from build123d import *

# Parameters (mm, degrees)
F0_W     = 30
F0_H     = 10
F0_R     = 2.75
F1_DEPTH = 7
F3_DEPTH = 15
F4_R     = 3
F5_R     = 1.5
F6_DEPTH = 25


# Not quite as in the source:
# - a feature names something its author has since deleted; it is built from what else it names


with BuildPart() as f1:
    # F0 (on Top) → F1 (new body)
    with BuildSketch(Plane.XY):
        with Locations((-23.3256115019, 35.3867347538)):
            Rectangle(F0_W, F0_H)
        with Locations((-32.3030129075, 35.3867347538)):
            Circle(F0_R, mode=Mode.SUBTRACT)
    extrude(amount=F1_DEPTH)

    # F2 (on face) → F3 (join)
    with BuildSketch(Plane.YZ.offset(-8.3256115019)):
        Polygon((30.3867347538, -10), (40.3867347538, 0), (30.3867347538, 0), align=None)
        Polygon((40.3867347538, 7), (40.3867347538, 0), (47.3867347538, 7), align=None)
    extrude(amount=-F3_DEPTH)

    # F4
    f4_edges = [f1.edges().sort_by_distance(p)[0] for p in [
        (-38.325612, 40.386735, 3.5),
        (-38.325612, 30.386735, 3.5),
    ]]
    fillet(f4_edges, radius=F4_R)

    # F5 (on face) → F6 (cut)
    with BuildSketch(Plane(origin=(0, 20.1933673769, -20.1933673769), x_dir=(1, 0, 0), z_dir=(0, 0.7071067812, -0.7071067812))):
        with Locations((-15.8256115019, -35.0243411958)):
            Circle(F5_R)
    extrude(amount=-F6_DEPTH, mode=Mode.SUBTRACT)


solid = f1.part
Geometry check sheet. Reference: the model listing, model coordinates, mm. A direction names the side the tool comes from. Give positions to 0.01 mm unless a question says otherwise; leave off trailing zeros. Order: outer loops, then holes, each group sorted by start corner. A loop starts at its lowest first (then second) coordinate and runs counter-clockwise, first axis right, second up. Notation, with made-up numbers: (40.5, 17) - (78.5, 17) arc R16 ccw to (78.5, 38) - close; hole circle Ø8 at (-33.5, -35). An arc over 180 degrees is marked (long way). Answer as a JSON object with one key per item and string values.
(1) Cross-section at C-C (z = 1.25). Record the cut outline in (x, y), then the cut area to 3 significant figures.
Report:
{"outline": "(-38.33, 33.39) arc R3 ccw to (-35.33, 30.39) - (-8.33, 30.39) - (-8.33, 41.64) - (-23.33, 41.64) - (-23.33, 40.39) - (-35.33, 40.39) arc R3 ccw to (-38.33, 37.39) - close; hole circle Ø5.5 at (-32.3, 35.39)", "area": "291 mm^2"}
(2) Cross-section at A-A (y = 35). Record the cut outline in (x, z).
Report:
{"outline": "(-38.33, 0) - (-35.03, 0) - (-35.03, 7) - (-38.33, 7) - close; (-29.58, 0) - (-23.33, 0) - (-23.33, -5.39) - (-8.33, -5.39) - (-8.33, 7) - (-29.58, 7) - close"}
(3) Cross-section at B-B (x = -33). Record the cut outline in (y, z).
Report:
{"outline": "(30.39, 0) - (32.73, 0) - (32.73, 7) - (30.39, 7) - close; (38.05, 0) - (40.39, 0) - (40.39, 7) - (38.05, 7) - close"}
(4) Depth check by flat-ended pin: pin 1 Ø9 at (x, y) = (-32.3, 35.39) entering from -Z; pin 2 Ø7.5 at (x, z) = (-28, 2) entering from +Y; pin 3 Ø3.5 at (y, z) = (43.5, 2.5) entering from -X. Enter the tip coordinate at first touch or a pass-through.
Report:
{"pin 1": "z = 0", "pin 2": "y = 40.39", "pin 3": "x = -23.33"}
(5) Draft check along X on faces 1 (the cylindrical face through (-16.02, 42.57, 4.86)), 2 (the flat face through (-23.326, 34, -4)), 3 (the cylindrical face through (-35.05, 35.51, 3.45)), 4 (the flat face through (-15.721, 38.768, -1.619)). Enter one of: released by +X, released by -X, zero draft, split by the parting line, or undercut.
Report:
{"face 1": "undercut", "face 2": "released by -X", "face 3": "undercut", "face 4": "zero draft"}
(6) Cross-section at D-D (x = -23.75). Record the cut outline in (y, z), then the cut area to 3 significant figures.
Report:
{"outline": "(30.39, 0) - (40.39, 0) - (40.39, 7) - (30.39, 7) - close", "area": "70.0 mm^2"}
(7) Material ranges on line 1 (X direction, y = 34.5, z = -4.5); line 2 (Z direction, x = -35.25, y = 39.75); line 3 (Y direction, x = -28.75, z = 5.5), recorded low to high.
Report:
{"line 1": "-23.33 to -8.33", "line 2": "0 to 7", "line 3": "30.39 to 40.39"}
(8) Tool access check on faces 5 (the flat face through (-20, 37, 7)), 6 (the flat face through (-29, 35, 0)), 7 (the flat face through (-23.326, 43, 4)). Record the directions out of +Z, -Z, +X, -X, +Y, -Y that give a thin tool (end or side, any length) a straight path to the whole face; none if there is none.
Report:
{"face 5": "+Z, +X, -X, +Y, -Y", "face 6": "-Z, -X, +Y, -Y", "face 7": "+Z, -Z, -X, +Y"}
